Source: CAD feature listing. Evaluate the final solid. Frame: model axes, mm. Round coordinates to 2 decimals unless told otherwise and drop trailing zeros. Loops run counter-clockwise (first coordinate to the right, second up) from the corner with the lowest first, then second, coordinate; pieces in that order, holes last. Notation, with made-up numbers: (8.25, 74) - (37.25, 74) arc R27 cw to (37.25, 96) - close; hole circle Ø4 at (-25.75, 22.25). An arc over 180 degrees is marked (long way). One line per question, with ' | ' between items. Start each with the question number.
1. Mould query, pull axis Y, two halves, no side actions, for faces 1 (the flat face through (-7.83, 26.36, 54.65)), 2 (the flat face through (8.244, -26.361, 63.296)), 3 (the flat face through (-1, 0, 51.827)). Classes: pulls with the +Y half, pulls with the -Y half, needs draft (parallel to the pull), parting line crosses it, or undercut.
2. Cut plane B-B (y = 15). Return loops of the section in (x, z) (3 decimals).
3. Cut plane C-C (z = 60.75). Return loops of the section in (x, y).
4. Cut plane A-A (x = 0). Return loops of the section in (y, z), then the cut area to 3 significant figures.
5. Cut plane D-D (z = 67). Return loops of the section in (x, y).
6. Pin query (flat end, axial travel): pin 1 (5 mm diameter, centred on y = -9.5, z = 64, fed in from -X); pin 2 (12 mm diameter, centred on y = 5.5, z = 62, fed in from +X); pin 3 (1 mm diameter, centred on y = 20, z = 68.5, fed in from -X). Return the tip coordinate at first contact, or that it passes through.
7. Ray query, line 1 (X direction, y = 12.5, z = 63.25); line 2 (X direction, y = 3, z = 63.5); line 3 (Z direction, x = -5.5, y = 1). Return the intervals inside material, ascending.
```python
from build123d import *
from OCP.BRepFilletAPI import BRepFilletAPI_MakeChamfer

# Parameters (mm, degrees)
SKETCH1_R           = 3.175
BOSS_EXTRUDE1_DEPTH = 53.975
CHAMFER1_SIZE       = 3.175
CHAMFER1_SIZE2      = 4.631063529
CHAMFER2_SIZE       = 1.27
CHAMFER2_SIZE2      = 2.749716278
CHAMFER2_SIZE2_2    = 2.199704526


# Read off the part's stored shape, not the designer's step: Imported1
with BuildPart() as part:
    # Sketch1 → Boss-Extrude1 (new body)
    with BuildSketch(Plane(origin=(0, -26.9875, 0), x_dir=(-1, 0, 0), z_dir=(0, -1, 0))):
        Polygon((-8.155551794, -74.05198332), (8.155551794, -74.05198332), (10.657362253, -51.82698332), (-10.657362253, -51.82698332), align=None)
        with Locations(Location((0, -61.35198332, 0), (0, 0, 270))):
            Circle(SKETCH1_R, mode=Mode.SUBTRACT)
    extrude(amount=-BOSS_EXTRUDE1_DEPTH)

    # Chamfer1: one chamfer whose edges measure the first distance from different faces: ONE call of the kernel's chamfer builder (chamfer() names one face for all edges)
    chamfer1_edges_1 = [part.edges().sort_by_distance(p)[0] for p in [
        (-10.657362253, 0, 51.82698332),
    ]]
    chamfer1_side_1 = [part.faces().sort_by_distance(p)[0] for p in [
        (0, 0, 51.82698332),
    ]]
    chamfer1_edges_2 = [part.edges().sort_by_distance(p)[0] for p in [
        (10.657362253, 0, 51.82698332),
    ]]
    chamfer1_side_2 = [part.faces().sort_by_distance(p)[0] for p in [
        (9.406457023, 0, 62.93948332),
    ]]
    chamfer1 = BRepFilletAPI_MakeChamfer(part.part.solid().wrapped)
    for e in chamfer1_edges_1:
        chamfer1.Add(CHAMFER1_SIZE, CHAMFER1_SIZE2, e.wrapped, chamfer1_side_1[0].wrapped)  # the first distance lies on this face
    for e in chamfer1_edges_2:
        chamfer1.Add(CHAMFER1_SIZE, CHAMFER1_SIZE2, e.wrapped, chamfer1_side_2[0].wrapped)  # the first distance lies on this face
    add(Compound.cast(chamfer1.Shape()), mode=Mode.REPLACE)

    # Chamfer2: one chamfer whose edges measure the first distance from different faces: ONE call of the kernel's chamfer builder (chamfer() names one face for all edges)
    chamfer2_edges_1 = [part.edges().sort_by_distance(p)[0] for p in [
        (8.155551794, 0, 74.05198332),
    ]]
    chamfer2_side_1 = [part.faces().sort_by_distance(p)[0] for p in [
        (0, 0, 74.05198332),
    ]]
    chamfer2_edges_2 = [part.edges().sort_by_distance(p)[0] for p in [
        (-9.147439527, -26.9875, 65.240482514),
        (-9.147439527, 26.9875, 65.240482514),
    ]]
    chamfer2_side_2 = [part.faces().sort_by_distance(p)[0] for p in [
        (-9.147439527, 0, 65.240482514),
    ]]
    chamfer2_edges_3 = [part.edges().sort_by_distance(p)[0] for p in [
        (0, -26.9875, 74.05198332),
        (0, 26.9875, 74.05198332),
    ]]
    chamfer2_side_3 = [part.faces().sort_by_distance(p)[0] for p in [
        (0, 0, 74.05198332),
    ]]
    chamfer2_edges_4 = [part.edges().sort_by_distance(p)[0] for p in [
        (9.228877825, 26.9875, 64.517019969),
        (9.228877825, -26.9875, 64.517019969),
    ]]
    chamfer2_side_4 = [part.faces().sort_by_distance(p)[0] for p in [
        (9.228877825, 0, 64.517019969),
    ]]
    chamfer2_edges_5 = [part.edges().sort_by_distance(p)[0] for p in [
        (-8.155551794, 0, 74.05198332),
    ]]
    chamfer2_side_5 = [part.faces().sort_by_distance(p)[0] for p in [
        (-9.147439527, 0, 65.240482514),
    ]]
    chamfer2_edges_6 = [part.edges().sort_by_distance(p)[0] for p in [
        (-0.728031765, -26.9875, 51.82698332),
        (-0.728031765, 26.9875, 51.82698332),
    ]]
    chamfer2_side_6 = [part.faces().sort_by_distance(p)[0] for p in [
        (-0.728031765, 0, 51.82698332),
    ]]
    chamfer2_edges_7 = [part.edges().sort_by_distance(p)[0] for p in [
        (8.16425129, -26.9875, 53.404519969),
        (8.16425129, 26.9875, 53.404519969),
    ]]
    chamfer2_side_7 = [part.faces().sort_by_distance(p)[0] for p in [
        (8.16425129, 0, 53.404519969),
    ]]
    chamfer2_edges_8 = [part.edges().sort_by_distance(p)[0] for p in [
        (-8.810844757, -26.9875, 54.127982514),
        (-8.810844757, 26.9875, 54.127982514),
    ]]
    chamfer2_side_8 = [part.faces().sort_by_distance(p)[0] for p in [
        (-8.810844757, 0, 54.127982514),
    ]]
    chamfer2 = BRepFilletAPI_MakeChamfer(part.part.solid().wrapped)
    for e in chamfer2_edges_1:
        chamfer2.Add(CHAMFER2_SIZE, CHAMFER2_SIZE2, e.wrapped, chamfer2_side_1[0].wrapped)  # the first distance lies on this face
    for e in chamfer2_edges_2:
        chamfer2.Add(CHAMFER2_SIZE, CHAMFER2_SIZE2_2, e.wrapped, chamfer2_side_2[0].wrapped)  # the first distance lies on this face
    for e in chamfer2_edges_3:
        chamfer2.Add(CHAMFER2_SIZE, CHAMFER2_SIZE2_2, e.wrapped, chamfer2_side_3[0].wrapped)  # the first distance lies on this face
    for e in chamfer2_edges_4:
        chamfer2.Add(CHAMFER2_SIZE, CHAMFER2_SIZE2_2, e.wrapped, chamfer2_side_4[0].wrapped)  # the first distance lies on this face
    for e in chamfer2_edges_5:
        chamfer2.Add(CHAMFER2_SIZE, CHAMFER2_SIZE2, e.wrapped, chamfer2_side_5[0].wrapped)  # the first distance lies on this face
    for e in chamfer2_edges_6:
        chamfer2.Add(CHAMFER2_SIZE, CHAMFER2_SIZE2_2, e.wrapped, chamfer2_side_6[0].wrapped)  # the first distance lies on this face
    for e in chamfer2_edges_7:
        chamfer2.Add(CHAMFER2_SIZE, CHAMFER2_SIZE2_2, e.wrapped, chamfer2_side_7[0].wrapped)  # the first distance lies on this face
    for e in chamfer2_edges_8:
        chamfer2.Add(CHAMFER2_SIZE, CHAMFER2_SIZE2_2, e.wrapped, chamfer2_side_8[0].wrapped)  # the first distance lies on this face
    add(Compound.cast(chamfer2.Shape()), mode=Mode.REPLACE)


solid = part.part
```
Answers follow:
1) face 1: pulls with the +Y half | face 2: pulls with the -Y half | face 3: needs draft
2) outline: (-10.139, 56.429) - (-7.482, 51.827) - (6.026, 51.827) - (10.302, 54.982) - (8.463, 71.32) - (6.886, 74.052) - (-5.406, 74.052) - (-8.298, 72.79) - close; hole circle Ø6.35 at (0, 61.352)
3) outline: (-9.65, -25.72) - (-7.44, -26.99) - (-3.12, -26.99) - (-3.12, 26.99) - (-7.44, 26.99) - (-9.65, 25.72) - close; (3.12, -26.99) - (7.44, -26.99) - (9.65, -25.72) - (9.65, 25.72) - (7.44, 26.99) - (3.12, 26.99) - close
4) outline: (-26.99, 54.03) - (-25.72, 51.83) - (25.72, 51.83) - (26.99, 54.03) - (26.99, 58.18) - (-26.99, 58.18) - close; (-26.99, 64.53) - (26.99, 64.53) - (26.99, 71.85) - (25.72, 74.05) - (-25.72, 74.05) - (-26.99, 71.85) - close | area: 851 mm2
5) outline: (-8.95, -25.72) - (-6.74, -26.99) - (6.74, -26.99) - (8.95, -25.72) - (8.95, 25.72) - (6.74, 26.99) - (-6.74, 26.99) - (-8.95, 25.72) - close
6) pin 1: stops at x = -9.57 | pin 2: stops at x = 10.19 | pin 3: stops at x = -8.84
7) line 1: x = -9.37 to -2.55, 2.55 to 9.37 | line 2: x = -9.34 to -2.34, 2.34 to 9.34 | line 3: z = 51.83 to 74.01
